```python
from build123d import *

# Parameters (mm, degrees)
SKETCH1_R           = 15
BOSS_EXTRUDE1_DEPTH = 20
SKETCH3_R           = 35
BOSS_EXTRUDE3_DEPTH = 8
SKETCH4_R           = 4
CUT_EXTRUDE1_DEPTH  = 8
SKETCH5_R           = 11
CUT_EXTRUDE2_DEPTH  = 8
SKETCH6_R           = 2
CUT_EXTRUDE3_DEPTH  = 15
FILLET1_R           = 1


with BuildPart() as part:
    # Sketch1 → Boss-Extrude1 (new body)
    with BuildSketch(Plane.XY):
        Circle(SKETCH1_R)
    extrude(amount=BOSS_EXTRUDE1_DEPTH)

    # Sketch3 → Boss-Extrude3 (add)
    with BuildSketch(Plane(origin=(0, 0, 0), x_dir=(-1, 0, 0), z_dir=(0, 0, -1))):
        Circle(SKETCH3_R)
    extrude(amount=BOSS_EXTRUDE3_DEPTH)

    # Sketch4 → Cut-Extrude1 (cut)
    with BuildSketch(Plane(origin=(0, 0, -8), x_dir=(-1, 0, 0), z_dir=(0, 0, -1))):
        with Locations((0, 28)):
            Circle(SKETCH4_R)
        with Locations((24.248711306, 14)):
            Circle(SKETCH4_R)
        with Locations((24.248711306, -14)):
            Circle(SKETCH4_R)
        with Locations((0, -28)):
            Circle(SKETCH4_R)
        with Locations((-24.248711306, -14)):
            Circle(SKETCH4_R)
        with Locations((-24.248711306, 14)):
            Circle(SKETCH4_R)
    extrude(amount=-CUT_EXTRUDE1_DEPTH, mode=Mode.SUBTRACT)

    # Sketch5 → Cut-Extrude2 (cut)
    with BuildSketch(Plane(origin=(0, 0, -8), x_dir=(-1, 0, 0), z_dir=(0, 0, -1))):
        Circle(SKETCH5_R)
    extrude(amount=-CUT_EXTRUDE2_DEPTH, mode=Mode.SUBTRACT)

    # Sketch6 → Cut-Extrude3 (cut)
    with BuildSketch(Plane.XY.offset(20)):
        with Locations((6, 6)):
            Circle(SKETCH6_R)
        with Locations(Location((-6, 6, 0), (0, 0, 180))):
            Circle(SKETCH6_R)
        with Locations(Location((6, -6, 0), (0, 0, 180))):
            Circle(SKETCH6_R)
        with Locations((-6, -6)):
            Circle(SKETCH6_R)
    extrude(amount=-CUT_EXTRUDE3_DEPTH, mode=Mode.SUBTRACT)

    # Fillet1
    fillet1_edges = [part.edges().sort_by_distance(p)[0] for p in [
        (11, 0, 0),
    ]]
    fillet(fillet1_edges, radius=FILLET1_R)


solid = part.part
```
The listing builds one solid part. Answer for the finished solid, in the listing's coordinates (mm). A direction names the side the tool comes from. Give positions to 0.01 mm unless a question says otherwise; leave off trailing zeros. Loops run counter-clockwise (first coordinate to the right, second up) from the corner with the lowest first, then second, coordinate; pieces in that order, holes last. Notation, with made-up numbers: M 14,64.5 L 38,64.5 A10 cw 38,70.5 Z; hole C -19,82 d7. An arc over 180 degrees is marked long. One line per item, written item: value.
1. Section A-A on y = -28 is taken. Determine the outline of the cut face in (x, z), plus the area to 3 significant figures.
Found:
outline: M -21,-8 L -4,-8 L -4,0 L -21,0 Z; M 4,-8 L 21,-8 L 21,0 L 4,0 Z
area: 272 mm^2
2. For faces 4 (the face through (8, 8, -8)), 5 (the face through (0, 0, 0)), 6 (the face through (-7.6, -7.2, 12.6)), determine the directions among +Z, -Z, +X, -X, +Y, -Y from which every point of the face is accessible in a straight line to the end or side of a thin tool.
Found:
face 4: -Z, +X, -X, +Y, -Y
face 5: -Z
face 6: +Z
3. Each of these flat-tipped pins is pushed along its axis until it touches: P1, Ø4.5, axis at x = -6, y = -6, coming from the -Z side; P2, Ø2, axis at x = 5.5, y = -5.5, coming from the +Z side; P3, Ø12, axis at y = -25, z = -5, coming from the -X side; P4, Ø6.5, axis at x = 0, y = 28, coming from the -Z side. Where does it stop, or does it pass through?
Found:
P1: z = -0.32
P2: z = 5
P3: x = -29.39
P4: through
4. Section B-B on z = -2.25 is taken. Determine the outline of the cut face in (x, y), plus the area to 3 significant figures.
Found:
outline: C 0,0 d70; hole C -24.25,-14 d8; hole C -24.25,14 d8; hole C 0,0 d22; hole C 0,-28 d8; hole C 0,28 d8; hole C 24.25,-14 d8; hole C 24.25,14 d8
area: 3,170 mm^2
5. Section D-D on x = 12.5 is taken. Determine the outline of the cut face in (y, z), plus the area to 3 significant figures.
Found:
outline: M -32.69,-8 L 32.69,-8 L 32.69,0 L 8.29,0 L 8.29,20 L -8.29,20 L -8.29,0 L -32.69,0 Z
area: 855 mm^2
6. Find the intervals of material crossed by probe 1 along X at (y, z) = (15, -1); probe 2 along Y at (x, z) = (-22.5, -1); probe 3 along Z at (x, y) = (-15.5, -19.5), in increasing order.
Found:
probe 1: -31.62 to -28.12, -20.38 to 20.38, 28.12 to 31.62
probe 2: -26.81 to -17.6, -10.4 to 10.4, 17.6 to 26.81
probe 3: -8 to 0
7. Section C-C on y = 13 is taken. Determine the outline of the cut face in (x, z).
Found:
outline: M -32.5,-8 L -28.12,-8 L -28.12,0 L -32.5,0 Z; M -20.38,-8 L 20.38,-8 L 20.38,0 L 7.48,0 L 7.48,20 L -7.48,20 L -7.48,0 L -20.38,0 Z; M 28.12,-8 L 32.5,-8 L 32.5,0 L 28.12,0 Z
8. For a pull along Y with two mould halves and no side action, classify faces 1 (the face through (6, -6, 5)), 2 (the face through (-15, -7, 0)), 3 (the face through (-14.985, 0.66, 9.86)) as pulls with the +Y half, pulls with the -Y half, needs draft (parallel to the pull), parting line crosses it, or undercut.
Found:
face 1: undercut
face 2: needs draft
face 3: parting line crosses it
